Geometry: final body of the model. Coordinates: model frame, mm. Face numbers are marked on the shaded views. A direction names the side the tool comes from. Round coordinates to 2 decimals unless told otherwise and drop trailing zeros. Write each loop counter-clockwise with the first axis right and the second up, starting at its lowest first coordinate (ties: lowest second). Pieces come first, ordered by that corner, then holes. Notation, with made-up numbers: M -4.75,81 L 52.25,81 A21 ccw 52.25,117 Z; hole C 89,27.5 d6. An arc over 180 degrees is marked long. Use one line per item in the form item = value. Start each with the question number.
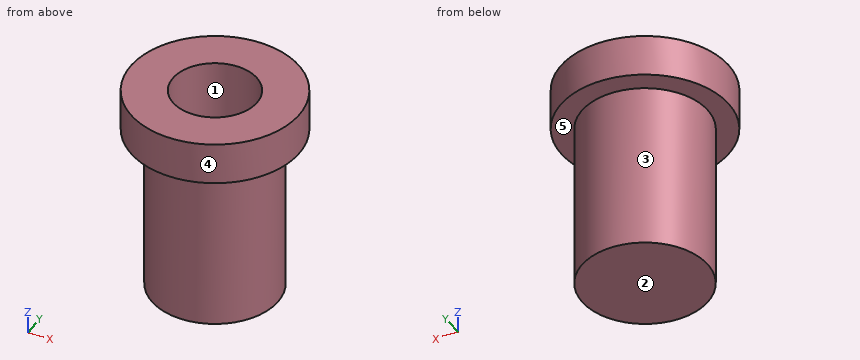
from build123d import *

# Parameters (mm, degrees)
SKETCH1_R           = 4
BOSS_EXTRUDE1_DEPTH = 2
SKETCH2_R           = 3
BOSS_EXTRUDE2_DEPTH = 8
SKETCH3_R           = 2
CUT_EXTRUDE1_DEPTH  = 8


with BuildPart() as part:
    # Sketch1 → Boss-Extrude1 (new body)
    with BuildSketch(Plane.XY):
        Circle(SKETCH1_R)
    extrude(amount=BOSS_EXTRUDE1_DEPTH)

    # Sketch2 → Boss-Extrude2 (add)
    with BuildSketch(Plane.XY):
        Circle(SKETCH2_R)
    extrude(amount=-BOSS_EXTRUDE2_DEPTH)

    # Sketch3 → Cut-Extrude1 (cut)
    with BuildSketch(Plane.XY.offset(2)):
        Circle(SKETCH3_R)
    extrude(amount=-CUT_EXTRUDE1_DEPTH, mode=Mode.SUBTRACT)


solid = part.part
1. Pull-direction query (Y, two-part tool) for the marked faces 1, 2 and 3; classes: released by +Y, released by -Y, zero draft, split by the parting line, or undercut.
2. Section query D-D (z = -7). Return loops of the section in (x, y).
3. Set-up query: the marked faces 4 and 5. Return all of +Z, -Z, +X, -X, +Y, -Y with unobstructed straight access to the full face (end or side cutting, diameter ignored); none if empty.
4. Section query A-A (y = 0). Return loops of the section in (x, z), then the cut area to 3 significant figures.
5. Ray query, probe 1 along Y at (x, z) = (0, -4); probe 2 along Z at (x, y) = (2.75, -1.5); probe 3 along Y at (x, z) = (-0.5, -5). Return the intervals inside material, ascending.
6. Contact query for flat-ended pins moving along their axis: pin 1 (2 mm diameter, centred on y = -2.5, z = 0.5, fed in from +X); pin 2 (1 mm diameter, centred on x = -2, z = -3, fed in from -Y); pin 3 (3 mm diameter, centred on x = 2.5, z = -1, fed in from +Y). Output: stop coordinate, or through.
7. Section query C-C (z = 0.5). Return loops of the section in (x, y), then the cut area to 3 significant figures.
Checks:
q1.face_1 = undercut
q1.face_2 = zero draft
q1.face_3 = split by the parting line
q2.outline = C 0,0 d6
q3.face_4 = +Z, -Z
q3.face_5 = -Z
q4.outline = M -4,0 L -3,0 L -3,-8 L 3,-8 L 3,0 L 4,0 L 4,2 L 2,2 L 2,-6 L -2,-6 L -2,2 L -4,2 Z
q4.area = 32.0 mm^2
q5.probe_1 = -3 to -2, 2 to 3
q5.probe_2 = 0 to 2
q5.probe_3 = -2.96 to -1.94, 1.94 to 2.96
q6.pin_1 = 3.71
q6.pin_2 = -2.6
q6.pin_3 = 3.75
q7.outline = C 0,0 d8; hole C 0,0 d4
q7.area = 37.7 mm^2
